CAD build for the part. Positions are in the model's coordinates, mm. A direction names the side the tool comes from. Coordinates: 2 decimals unless noted, no trailing zeros. Loops run counter-clockwise (first coordinate to the right, second up) from the corner with the lowest first, then second, coordinate; pieces in that order, holes last.
1) Saw through at C-C, the plane y = 1.5. Write the cut outline in (x, z).
2) Saw through at A-A, the plane z = 5. Write the cut outline in (x, y).
3) Two-plate mould, pull along Y, no slides. Class faces 3 (the flat face through (25, 0, 5)), 4 (the cylindrical face through (-3, 0, 5)), 5 (the flat face through (-1, 4, 5)), 6 (the cylindrical face through (34.536, 2.028, 4.675)): +Y half, -Y half, draft (parallel to the pull), parting line (faces both ways), or undercut.
4) Wall check: line 1 along Y through (x, z) = (0, 3); line 2 along X through (y, z) = (-2.25, 7.25); line 3 along X through (y, z) = (2.05, 5). Give the ranges that are in metal, low to high.
5) Saw through at D-D, the plane z = 8.75. Write the cut outline in (x, y), and give its area (3 significant figures).
6) Pin check, flat tips, straight feed: pin 1 Ø5 at (x, y) = (25, -1) entering from +Z; pin 2 Ø1.8 at (x, z) = (-36, 5) entering from +Y; pin 3 Ø1.5 at (x, z) = (6, 7.5) entering from -Y; pin 4 Ø3 at (x, z) = (-26.5, 4.5) entering from -Y. Stop position of each tip, or through.
7) Which spindle directions (+Z, -Z, +X, -X, +Y, -Y) get a long thin tool onto all of the face, cutting with end or side? Do faces 1 (the flat face through (-25, 0, 5)), 2 (the flat face through (-40, 2, 5)). Say none if no direction does.
8) Saw through at B-B, the plane x = 0. Write the cut outline in (y, z).
```python
from build123d import *

# Parameters (mm, degrees)
ESQUISSE1_R             = 3
BOSS_EXTRU_1_DEPTH      = 10
ESQUISSE2_R             = 1.5
ENL_V_MAT_EXTRU_1_DEPTH = 44.543082114


with BuildPart() as part:
    # Esquisse1 → Boss.-Extru.1 (new body)
    with BuildSketch(Plane.XY):
        with BuildLine():
            Line((-10, 0), (-40, 0))
            Line((-40, 0), (-40, 4))
            Line((-40, 4), (40, 4))
            Line((40, 4), (40, 0))
            Line((40, 0), (10, 0))
            ThreePointArc((10, 0), (0, -10), (-10, 0))
        make_face()
        Circle(ESQUISSE1_R, mode=Mode.SUBTRACT)
    extrude(amount=BOSS_EXTRU_1_DEPTH)

    # Esquisse2 → Enlèv. mat.-Extru.1 (cut, through all)
    with BuildSketch(Plane(origin=(0, 4, 0), x_dir=(1, 0, 0), z_dir=(0, 1, 0))):
        with Locations(Location((-36, -5, 0), (0, 0, 270))):
            Circle(ESQUISSE2_R)
        with Locations(Location((36, -5, 0), (0, 0, 270))):
            Circle(ESQUISSE2_R)
    extrude(amount=-ENL_V_MAT_EXTRU_1_DEPTH, mode=Mode.SUBTRACT)


solid = part.part
```
Data:
1. outline: (-40, 0) - (-2.6, 0) - (-2.6, 10) - (-40, 10) - close; (2.6, 0) - (40, 0) - (40, 10) - (2.6, 10) - close; hole circle Ø3 at (-36, 5); hole circle Ø3 at (36, 5)
2. outline: (-40, 0) - (-37.5, 0) - (-37.5, 4) - (-40, 4) - close; (-34.5, 0) - (-10, 0) arc R10 ccw to (10, 0) - (34.5, 0) - (34.5, 4) - (-34.5, 4) - close; (37.5, 0) - (40, 0) - (40, 4) - (37.5, 4) - close; hole circle Ø6 at (0, 0)
3. face 3: -Y half
3. face 4: undercut
3. face 5: +Y half
3. face 6: draft
4. line 1: y = -10 to -3, 3 to 4
4. line 2: x = -9.74 to -1.98, 1.98 to 9.74
4. line 3: x = -40 to -37.5, -34.5 to -2.19, 2.19 to 34.5, 37.5 to 40
5. outline: (-40, 0) - (-10, 0) arc R10 ccw to (10, 0) - (40, 0) - (40, 4) - (-40, 4) - close; hole circle Ø6 at (0, 0)
5. area: 449 mm2
6. pin 1: stops at z = 10
6. pin 2: passes through
6. pin 3: stops at y = -8.51
6. pin 4: stops at y = 0
7. face 1: +Z, -Z, -X, -Y
7. face 2: +Z, -Z, -X, +Y, -Y
8. outline: (-10, 0) - (-3, 0) - (-3, 10) - (-10, 10) - close; (3, 0) - (4, 0) - (4, 10) - (3, 10) - close
